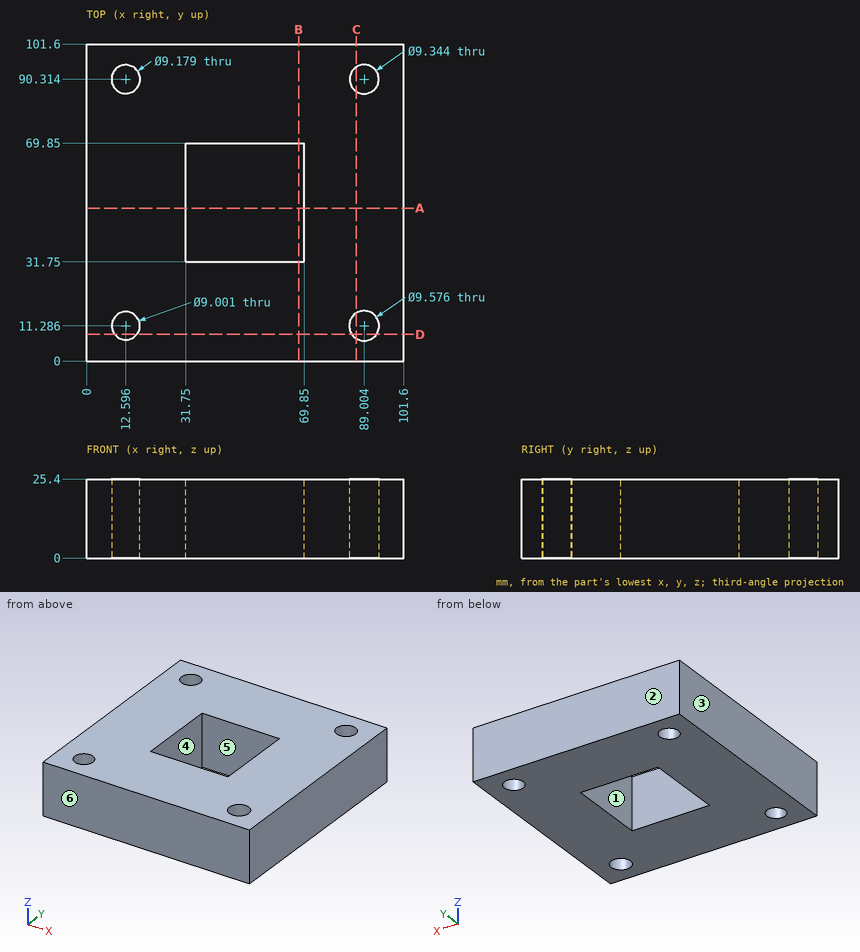
Study the drawing (mm; zero at the part's minimum x, y, z) and answer. A direction names the side the tool comes from. Coordinates: 2 decimals unless noted, no trailing zeros. Write each loop counter-clockwise with the first axis right and the second up, starting at its lowest first coordinate (ties: lowest second). Pieces come first, ordered by that corner, then holes.
Q1. Section C-C, the plane x = 86.5 is taken. Write down the section's boundary in (y, z) (1 decimal), then the cut area to 3 significant figures.
Returned:
outline: (0, 0) - (7.2, 0) - (7.2, 25.4) - (0, 25.4) - close; (15.4, 0) - (86.4, 0) - (86.4, 25.4) - (15.4, 25.4) - close; (94.3, 0) - (101.6, 0) - (101.6, 25.4) - (94.3, 25.4) - close
area: 2,170 mm2
Q2. The mould has two halves that part along Y. Classify the marked faces 1, 2, 3 and 4: released by +Y, released by -Y, zero draft, split by the parting line, or undercut.
Returned:
face 1: undercut
face 2: released by +Y
face 3: zero draft
face 4: undercut
Q3. Section A-A, the plane y = 49 is taken. Write down the section's boundary in (x, z), then the cut area to 3 significant figures.
Returned:
outline: (0, 0) - (31.75, 0) - (31.75, 25.4) - (0, 25.4) - close; (69.85, 0) - (101.6, 0) - (101.6, 25.4) - (69.85, 25.4) - close
area: 1,610 mm2
Q4. Find the intervals of material crossed by line 1 along X through (y, z) = (46, 23.75); line 2 along Y through (x, z) = (11.5, 14), in increasing order.
Returned:
line 1: x = 0 to 31.75, 69.85 to 101.6
line 2: y = 0 to 6.92, 15.65 to 85.86, 94.77 to 101.6
Q5. Section D-D, the plane y = 8.5 is taken. Write down the section's boundary in (x, z), then the cut area to 3 significant figures.
Returned:
outline: (0, 0) - (9.06, 0) - (9.06, 25.4) - (0, 25.4) - close; (16.13, 0) - (85.11, 0) - (85.11, 25.4) - (16.13, 25.4) - close; (92.9, 0) - (101.6, 0) - (101.6, 25.4) - (92.9, 25.4) - close
area: 2,200 mm2
Q6. Which of the six approach directions +Z, -Z, +X, -X, +Y, -Y give full straight-line access (tool end or side, diameter ignored) to the marked faces 5 and 6?
Returned:
face 5: +Z, -Z
face 6: +Z, -Z, +X, -X, -Y
